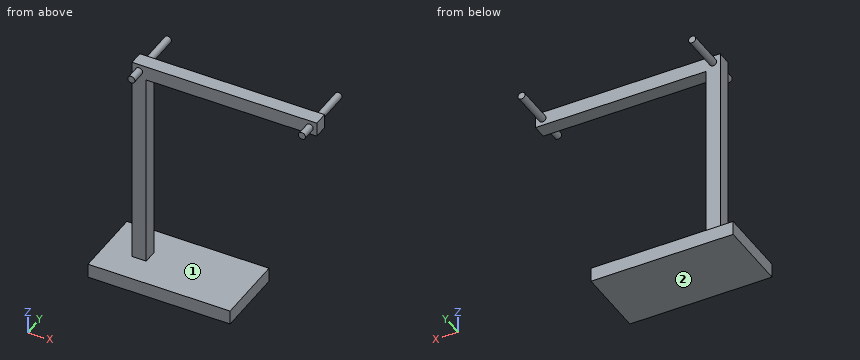
from build123d import *

# Parameters (mm, degrees)
SKETCH1_W           = 100
SKETCH1_H           = 50
BOSS_EXTRUDE1_DEPTH = 10
SKETCH2_W           = 10
SKETCH2_H           = 10
BOSS_EXTRUDE2_DEPTH = 150
SKETCH3_W           = 10
SKETCH3_H           = 10
BOSS_EXTRUDE3_DEPTH = 120
SKETCH4_R           = 2.5
BOSS_EXTRUDE4_DEPTH = 10
BOSS_EXTRUDE5_START = -27
SKETCH5_R           = 2.5
BOSS_EXTRUDE5_DEPTH = 27


with BuildPart() as part:
    # Sketch1 → Boss-Extrude1 (new body)
    with BuildSketch(Plane.XY):
        Rectangle(SKETCH1_W, SKETCH1_H)
    extrude(amount=BOSS_EXTRUDE1_DEPTH)

    # Sketch2 → Boss-Extrude2 (add)
    with BuildSketch(Plane.XY.offset(10)):
        with Locations((-25, 0)):
            Rectangle(SKETCH2_W, SKETCH2_H)
    extrude(amount=BOSS_EXTRUDE2_DEPTH)

    # Sketch3 → Boss-Extrude3 (add)
    with BuildSketch(Plane(origin=(-20, 0, 0), x_dir=(0, 0, -1), z_dir=(1, 0, 0))):
        with Locations((-155, 0)):
            Rectangle(SKETCH3_W, SKETCH3_H)
    extrude(amount=BOSS_EXTRUDE3_DEPTH)

    # Sketch4 → Boss-Extrude4 (add)
    with BuildSketch(Plane.XZ.offset(5)):
        with Locations(Location((-25, 155, 0), (0, 0, 180))):
            Circle(SKETCH4_R)
        with Locations(Location((95, 155, 0), (0, 0, 180))):
            Circle(SKETCH4_R)
    extrude(amount=BOSS_EXTRUDE4_DEPTH)

    # Sketch5 → Boss-Extrude5 (add)
    with BuildSketch(Plane(origin=(0, 5, -5), x_dir=(-1, 0, 0), z_dir=(0, -1, 0)).offset(BOSS_EXTRUDE5_START)):
        with Locations((-95, -160)):
            Circle(SKETCH5_R)
        with Locations((25, -160)):
            Circle(SKETCH5_R)
    extrude(amount=BOSS_EXTRUDE5_DEPTH)


solid = part.part
Read the model definition and answer for the solid it produces. Units are mm, in the model's axes. Face numbers are marked on the shaded views. Coordinates: 2 decimals unless noted, no trailing zeros. Order: outer loops, then holes, each group sorted by start corner. A loop starts at its lowest first (then second) coordinate and runs counter-clockwise, first axis right, second up. Notation, with made-up numbers: (36, 82) -> (55, 82) arc R37 ccw to (55, 120) -> close; hole circle Ø8 at (56, 35). An arc over 180 degrees is marked (long way). Answer as a JSON object with one key per item and string values.
1) Consider line 1 along Z through (x, y) = (-6.5, -15.5); line 2 along Z through (x, y) = (8, 0.5); line 3 along Y through (x, z) = (24.5, 150.5). Determine where each line is inside the solid, lowest interval first. Write a range as from..to.
Model answer:
{"line 1": "z = 0..10", "line 2": "z = 0..10, 150..160", "line 3": "y = -5..5"}
2) The mould has two halves that part along Z. Classify the marked faces 1 and 2: released by +Z, released by -Z, zero draft, split by the parting line, or undercut.
Model answer:
{"face 1": "undercut", "face 2": "released by -Z"}
3) A cutting plane is placed at C-C, the plane x = -25. Determine the outline of the cut face in (y, z).
Model answer:
{"outline": "(-25, 0) -> (25, 0) -> (25, 10) -> (5, 10) -> (5, 152.5) -> (32, 152.5) -> (32, 157.5) -> (5, 157.5) -> (5, 160) -> (-5, 160) -> (-5, 157.5) -> (-15, 157.5) -> (-15, 152.5) -> (-5, 152.5) -> (-5, 10) -> (-25, 10) -> close"}
4) Each of these flat-tipped pins is pushed along its axis until it touches: pin 1 (5 mm diameter, centred on y = 1.5, z = 111.5, fed in from +X); pin 2 (5.5 mm diameter, centred on x = -25.5, z = 155.5, fed in from -Y); pin 3 (11 mm diameter, centred on y = -12, z = 5, fed in from +X). Where does it stop, or does it pass through?
Model answer:
{"pin 1": "stops at x = -20", "pin 2": "stops at y = -15", "pin 3": "stops at x = 50"}
5) A cutting plane is placed at B-B, the plane y = -11. Determine the outline of the cut face in (x, z).
Model answer:
{"outline": "(-50, 0) -> (50, 0) -> (50, 10) -> (-50, 10) -> close; circle Ø5 at (-25, 155); circle Ø5 at (95, 155)"}
6) A cutting plane is placed at A-A, the plane x = 16. Determine the outline of the cut face in (y, z).
Model answer:
{"outline": "(-25, 0) -> (25, 0) -> (25, 10) -> (-25, 10) -> close; (-5, 150) -> (5, 150) -> (5, 160) -> (-5, 160) -> close"}
7) A cutting plane is placed at D-D, the plane z = 155. Determine the outline of the cut face in (x, y), plus the area to 3 significant figures.
Model answer:
{"outline": "(-30, -5) -> (-27.5, -5) -> (-27.5, -15) -> (-22.5, -15) -> (-22.5, -5) -> (92.5, -5) -> (92.5, -15) -> (97.5, -15) -> (97.5, -5) -> (100, -5) -> (100, 5) -> (97.5, 5) -> (97.5, 32) -> (92.5, 32) -> (92.5, 5) -> (-22.5, 5) -> (-22.5, 32) -> (-27.5, 32) -> (-27.5, 5) -> (-30, 5) -> close", "area": "1,670 mm²"}
